Autodesk Inventor part; units mm, degrees
ref_plane "YZ Plane" through (0, 0, 0) normal (1, 0, 0) x (0, 1, 0)
ref_plane "XZ Plane" through (0, 0, 0) normal (0, 1, 0) x (-1, 0, 0)
ref_plane "XY Plane" through (0, 0, 0) normal (0, 0, 1) x (1, 0, 0)
sketch "Sketch1" plane through (0, 0, 0) normal (0, 1, 0) x (-1, 0, 0)
  line L0 (0, 0) -> (50.8, 0)
  line L1 (50.8, 0) -> (50.8, -25.4)
  line L2 (50.8, -25.4) -> (0, -25.4)
  line L3 (0, -25.4) -> (0, 0)
  dimension "d0" = 25.4
  dimension "d1" = 50.8
extrude "Extrusion1" add sketch "Sketch1" along normal blind 31.75
sketch "Sketch3" plane through (0, 0, 0) normal (1, 0, 0) x (0, 0, -1)
  circle A0 centre (12.7, 25.4) radius 2.581
  line L0 (0, 31.75) -> (25.4, 31.75)
  circle A1 centre (12.7, 6.35) radius 2.3807
  point P0 (0, 0)
  dimension "d6" = 6.35
  dimension "d7" = 19.05
hole "Hole1" at (0, 25.4, -12.7) at (0, 6.35, -12.7) direction (-1, 0, 0) diameter 5.3594 depth 17.2466 tip angle 118
sketch "Sketch4" plane through (0, 31.75, 0) normal (0, 1, 0) x (1, 0, 0)
  line L0 (0, 0) -> (0, 25.4)
  line L1 (0, 12.7) -> (146.05, 12.7) construction
  circle A0 centre (146.05, 12.7) radius 147.32
  dimension "d15" = 146.05
  dimension "d16" = 294.64
extrude "Extrusion2" cut sketch "Sketch4" against normal blind 50.8
sketch "Sketch6" plane through (0, 0, 0) normal (0, -1, 0) x (1, 0, 0)
  circle A0 centre (-44.45, -12.7) radius 4.2294
  line L0 (-0.7216, 0) -> (-50.8, 0)
  line L1 (-50.8, 0) -> (-50.8, -25.4)
  circle A1 centre (-25.4, -12.7) radius 3.8351
  point P0 (0, 0)
  dimension "d21" = 12.7
  dimension "d22" = 6.35
  dimension "d23" = 19.05
hole "Hole2" at (-44.45, 0, -12.7) at (-25.4, 0, -12.7) direction (0, 1, 0) diameter 5.3594 depth 17.2466 tip angle 118
properties part number "mountingStub" material "Aluminum 6061"
Geometry: final body of the model. Coordinates: model frame, mm. A direction names the side the tool comes from. Give positions to 0.01 mm unless a question says otherwise; leave off trailing zeros. Write each loop counter-clockwise with the first axis right and the second up, starting at its lowest first coordinate (ties: lowest second). Pieces come first, ordered by that corner, then holes. Notation, with made-up numbers: (78, 10.5) -> (121, 10.5) arc R12 cw to (121, 29.5) -> close; hole circle Ø8 at (-34.75, -24). An arc over 180 degrees is marked (long way). Answer as a JSON object with one key per item and string values.
1. Cut plane B-B on y = 16. Output: boundary loops of the cut face in (x, z), and give its area (3 significant figures).
Ans:
{"outline": "(-50.8, -25.4) -> (-0.72, -25.4) arc R147.32 cw to (-0.72, 0) -> (-50.8, 0) -> close; hole circle Ø5.36 at (-44.45, -12.7); hole circle Ø5.36 at (-25.4, -12.7)", "area": "1,220 mm^2"}
2. Cut plane A-A on x = -15.5. Output: boundary loops of the cut face in (y, z).
Ans:
{"outline": "(0, -25.4) -> (31.75, -25.4) -> (31.75, 0) -> (0, 0) -> close; hole circle Ø5.36 at (6.35, -12.7); hole circle Ø5.36 at (25.4, -12.7)"}
3. Ray query, probe 1 along Y at (x, z) = (-5, -12.7); probe 2 along X at (y, z) = (11.25, -12.7); probe 3 along Z at (x, y) = (-25.4, 8.25). Return the intervals inside material, ascending. Write a range as from..to.
Ans:
{"probe 1": "y = 0..3.67, 9.03..22.72, 28.08..31.75", "probe 2": "x = -50.8..-47.13, -41.77..-28.08, -22.72..-1.27", "probe 3": "z = -25.4..-15.38, -10.02..0"}
4. Contact query for flat-ended pins moving along their axis: pin 1 (4 mm diameter, centred on x = -42.5, z = -2.5, fed in from -Y); pin 2 (8.5 mm diameter, centred on y = 6.35, z = -12.7, fed in from +X); pin 3 (1.5 mm diameter, centred on y = 4, z = -7, fed in from +X); pin 4 (3 mm diameter, centred on y = 4, z = -3, fed in from +X). Output: stop coordinate, or through.
Ans:
{"pin 1": "stops at y = 0", "pin 2": "stops at x = -1.21", "pin 3": "stops at x = -1.13", "pin 4": "stops at x = -0.84"}
5. Mould query, pull axis Y, two halves, no side actions, for faces 1 (the cylindrical face through (-9.358, 7.376, -15.175)), 2 (the flat face through (-25.4, 0, -9.7)), 3 (the cylindrical face through (-9.358, 24.595, -15.256)), 4 (the cylindrical face through (-43.424, 8.744, -15.175)). Classes: pulls with the +Y half, pulls with the -Y half, needs draft (parallel to the pull), parting line crosses it, or undercut.
Ans:
{"face 1": "undercut", "face 2": "pulls with the -Y half", "face 3": "undercut", "face 4": "needs draft"}
6. Cut plane C-C on y = 5. Count the separate pieces of the cut face and the enclosed holes in it, and give its area (3 significant figures).
Ans:
{"separate pieces": "1", "enclosed holes": "2", "area": "1,140 mm^2"}
7. Access query for faces 5 (the conical face through (-18.58, 24.95, -12.6)), 6 (the cylindrical face through (-24.374, 8.744, -15.175)). Directions: +Z, -Z, +X, -X, +Y, -Y. A direction counts if a zero-diameter tool reaches every point of the face in a straight line with its end or side. Return the directions, or none.
Ans:
{"face 5": "+X", "face 6": "-Y"}
